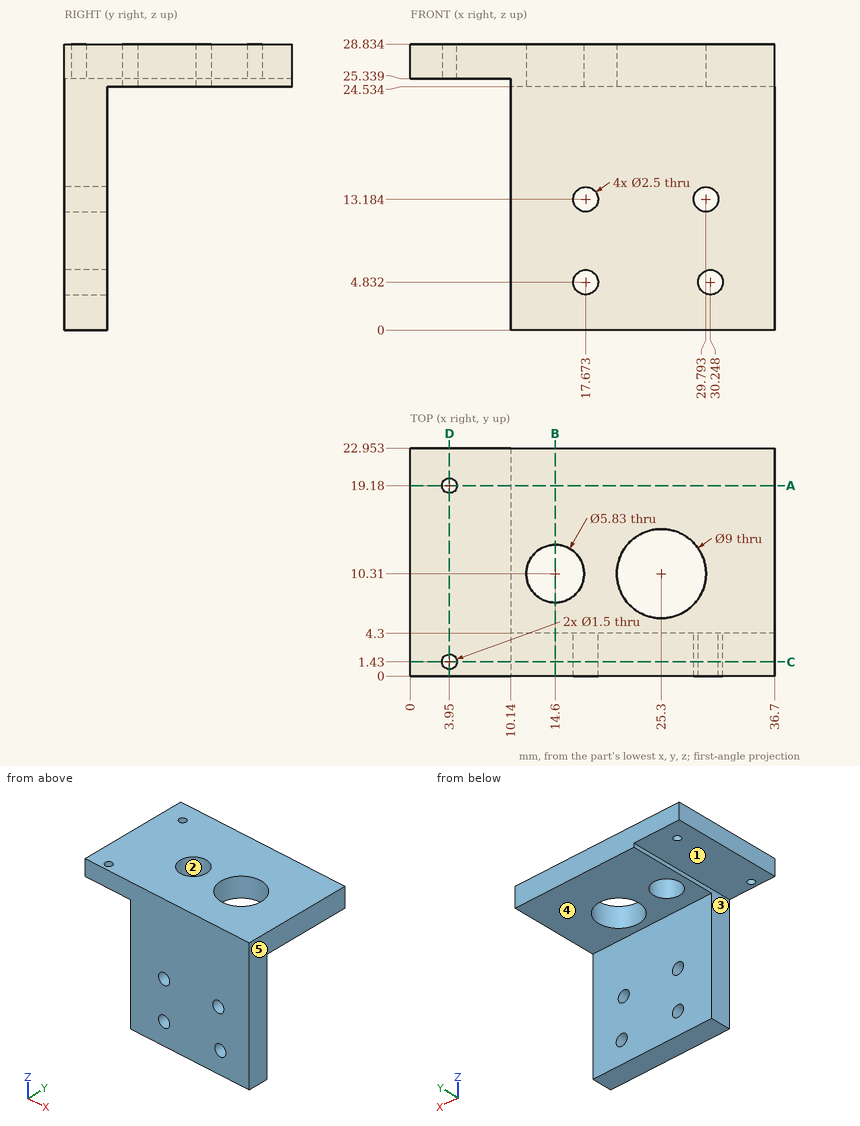
Source: three-view drawing plus pictorial views. Frame: mm from the lowest corner of the part. A direction names the side the tool comes from. Give positions to 0.01 mm unless a question says otherwise; leave off trailing zeros. Loops run counter-clockwise (first coordinate to the right, second up) from the corner with the lowest first, then second, coordinate; pieces in that order, holes last. Notation, with made-up numbers: (44.5, -14.5) -> (72.5, -14.5) arc R7 cw to (72.5, -1.5) -> close; hole circle Ø8 at (88, 42). An arc over 180 degrees is marked (long way). Use a Markdown table: item, result. Add a question column.
(1) Pull-direction query (X, two-part tool) for the marked faces 1, 2 and 3; classes: +X half, -X half, draft (parallel to the pull), parting line (faces both ways), or undercut.
(2) First-contact query: pin 1 Ø2.5 at (x, y) = (3.95, 1.43) entering from +Z; pin 2 Ø6.5 at (x, y) = (14.6, 10.31) entering from -Z; pin 3 Ø10 at (y, z) = (5.5, 13.5) entering from -X; pin 4 Ø7.5 at (x, z) = (28, 10) entering from +Y. Flat tips, straight axial feed; report the tip coordinate or a pass-through.
(3) Section query D-D (x = 3.95). Output: boundary loops of the cut face in (y, z) (1 decimal).
(4) Section query C-C (y = 1.43). Count the separate pieces of the cut face and the enclosed holes in it.
(5) Ray query, line 1 (Y direction, x = 25.3, z = 27.4); line 2 (X direction, y = 1.75, z = 14.25) (1 decimal); line 3 (Y direction, x = 3.95, z = 26.55). Return the intervals inside material, ascending.
(6) Section query A-A (y = 19.18). Output: boundary loops of the cut face in (x, z) (1 decimal).
(7) Section query B-B (x = 14.6). Output: boundary loops of the cut face in (y, z) (1 decimal).
(8) Access query for the marked faces 4 and 5. Directions: +Z, -Z, +X, -X, +Y, -Y. A direction counts if a zero-diameter tool reaches every point of the face in a straight line with its end or side. Return the directions, or none.
Checked values:
| question | item | result |
|---|---|---|
| 1 | face 1 | draft |
| 1 | face 2 | undercut |
| 1 | face 3 | -X half |
| 2 | pin 1 | z = 28.83 |
| 2 | pin 2 | z = 24.53 |
| 2 | pin 3 | x = 10.14 |
| 2 | pin 4 | y = 4.3 |
| 3 | outline | (0, 25.3) -> (0.7, 25.3) -> (0.7, 28.8) -> (0, 28.8) -> close; (2.2, 25.3) -> (18.4, 25.3) -> (18.4, 28.8) -> (2.2, 28.8) -> close; (19.9, 25.3) -> (23, 25.3) -> (23, 28.8) -> (19.9, 28.8) -> close |
| 4 | separate pieces | 2 |
| 4 | enclosed holes | 4 |
| 5 | line 1 | 0 to 5.81, 14.81 to 22.95 |
| 5 | line 2 | 10.1 to 17, 18.3 to 29.1, 30.4 to 36.7 |
| 5 | line 3 | 0 to 0.68, 2.18 to 18.43, 19.93 to 22.95 |
| 6 | outline | (0, 25.3) -> (3.2, 25.3) -> (3.2, 28.8) -> (0, 28.8) -> close; (4.7, 25.3) -> (10.1, 25.3) -> (10.1, 24.5) -> (36.7, 24.5) -> (36.7, 28.8) -> (4.7, 28.8) -> close |
| 7 | outline | (0, 0) -> (4.3, 0) -> (4.3, 24.5) -> (7.4, 24.5) -> (7.4, 28.8) -> (0, 28.8) -> close; (13.2, 24.5) -> (23, 24.5) -> (23, 28.8) -> (13.2, 28.8) -> close |
| 8 | face 4 | -Z, +X, -X, +Y |
| 8 | face 5 | +Z, -Z, +X, +Y, -Y |
